```python
from build123d import *

# Parameters (mm, degrees)
F0_W     = 63.14
F0_H     = 60.6
F1_DEPTH = 12.57
F2_W     = 47.4
F2_H     = 3.18
F3_DEPTH = 8.45
F5_W     = 2.59
F5_H     = 3.3
F6_DEPTH = 3.18


# Not quite as in the source:
# - a feature names something its author has since deleted; it is built from what else it names


with BuildPart() as f1:
    # F0 (on Top) → F1 (new body)
    with BuildSketch(Plane.XY):
        Rectangle(F0_W, F0_H)
    extrude(amount=F1_DEPTH)

    # F2 (on face) → F3 (join)
    with BuildSketch(Plane(origin=(-31.57, 0, 0), x_dir=(0, -1, 0), z_dir=(-1, 0, 0))):
        with Locations((0, 1.59)):
            Rectangle(F2_W, F2_H)
    extrude(amount=F3_DEPTH)

    # F4: F1 across plane


with BuildPart() as f1_1:
    add(f1.part)
    add(f1.part.mirror(Plane.YZ))

    # F5 (on face) → F6 (cut, through all)
    with BuildSketch(Plane.XY.offset(3.18)):
        with Locations((-38.725, 16.5)):
            Rectangle(F5_W, F5_H)
        with BuildLine():
            Line((-37.43, 18.15), (-37.43, 14.85))
            ThreePointArc((-37.43, 14.85), (-35.78, 16.5), (-37.43, 18.15))
        make_face()
        with Locations((-38.725, 0)):
            Rectangle(F5_W, F5_H)
        with BuildLine():
            ThreePointArc((-37.43, -1.65), (-35.78, 0), (-37.43, 1.65))
            Line((-37.43, 1.65), (-37.43, -1.65))
        make_face()
        with Locations((-38.725, -16.5)):
            Rectangle(F5_W, F5_H)
        with BuildLine():
            ThreePointArc((-37.43, -18.15), (-35.78, -16.5), (-37.43, -14.85))
            Line((-37.43, -14.85), (-37.43, -18.15))
        make_face()
        with BuildLine():
            Line((37.43, 14.85), (37.43, 18.15))
            ThreePointArc((37.43, 18.15), (35.78, 16.5), (37.43, 14.85))
        make_face()
        with Locations((38.725, 16.5)):
            Rectangle(F5_W, F5_H)
        with BuildLine():
            ThreePointArc((37.43, 1.65), (35.78, 0), (37.43, -1.65))
            Line((37.43, -1.65), (37.43, 1.65))
        make_face()
        with Locations((38.725, 0)):
            Rectangle(F5_W, F5_H)
        with BuildLine():
            ThreePointArc((37.43, -14.85), (35.78, -16.5), (37.43, -18.15))
            Line((37.43, -18.15), (37.43, -14.85))
        make_face()
        with Locations((38.725, -16.5)):
            Rectangle(F5_W, F5_H)
    extrude(amount=-F6_DEPTH, mode=Mode.SUBTRACT)


solid = f1_1.part
```
Input: part model. Units: mm. Frame: model coordinates. A direction names the side the tool comes from. Give positions to 0.01 mm unless a question says otherwise; leave off trailing zeros. Order: outer loops, then holes, each group sorted by start corner. A loop starts at its lowest first (then second) coordinate and runs counter-clockwise, first axis right, second up.
1. Pin query (flat end, axial travel): pin 1 Ø4 at (y, z) = (2, 4.5) entering from -X; pin 2 Ø3 at (x, z) = (39, 1) entering from -Y; pin 3 Ø6.5 at (y, z) = (0, 9) entering from +X; pin 4 Ø4 at (x, y) = (37, 10) entering from +Z. Return the tip coordinate at first contact, or that it passes through.
Computed:
pin 1: stops at x = -40.02
pin 2: stops at y = -23.7
pin 3: stops at x = 31.57
pin 4: stops at z = 3.18
2. Cut plane C-C (y = 16.5). Return loops of the section in (x, z), and give its area (3 significant figures).
Computed:
outline: (-35.78, 0) - (35.78, 0) - (35.78, 3.18) - (31.57, 3.18) - (31.57, 12.57) - (-31.57, 12.57) - (-31.57, 3.18) - (-35.78, 3.18) - close
area: 820 mm2
3. Set-up query: faces 1 (the face through (36, 23.7, 2)), 2 (the face through (-39, -14.85, 2)), 3 (the face through (-35, 0, 3.18)), 4 (the face through (39, 1.65, 2)), 5 (the face through (36, -23.7, 2)). Return all of +Z, -Z, +X, -X, +Y, -Y with unobstructed straight access to the full face (end or side cutting, diameter ignored); none if empty.
Computed:
face 1: +Z, -Z, +X, +Y
face 2: +Z, -Z, -X
face 3: +Z, -X, +Y, -Y
face 4: +Z, -Z, +X
face 5: +Z, -Z, +X, -Y
4. Cut plane A-A (y = 4). Return loops of the section in (x, z).
Computed:
outline: (-40.02, 0) - (40.02, 0) - (40.02, 3.18) - (31.57, 3.18) - (31.57, 12.57) - (-31.57, 12.57) - (-31.57, 3.18) - (-40.02, 3.18) - close
5. Cut plane B-B (z = 8). Return loops of the section in (x, y).
Computed:
outline: (-31.57, -30.3) - (31.57, -30.3) - (31.57, 30.3) - (-31.57, 30.3) - close
6. Line query: probe 1 along X at (y, z) = (15.5, 5.75); probe 2 along Z at (x, y) = (35.5, -15.5). Output: solid intervals per line, ascending.
Computed:
probe 1: x = -31.57 to 31.57
probe 2: z = 0 to 3.18
